Input: part model. Units: mm. Frame: model coordinates. A direction names the side the tool comes from. Round coordinates to 2 decimals unless told otherwise and drop trailing zeros. Loops run counter-clockwise (first coordinate to the right, second up) from the corner with the lowest first, then second, coordinate; pieces in that order, holes last.
(1) Access query for faces 4 (the face through (2, 40, -30)), 5 (the face through (2, 50, -10)), 6 (the face through (2, 3, -20)). Directions: +Z, -Z, +X, -X, +Y, -Y. A direction counts if a zero-diameter tool reaches every point of the face in a straight line with its end or side. Return the directions, or none.
(2) Cut plane D-D, the plane y = 13. Output: boundary loops of the cut face in (x, z), and give its area (3 significant figures).
(3) Cut plane C-C, the plane z = -85. Output: boundary loops of the cut face in (x, y), and give its area (3 significant figures).
(4) Cut plane B-B, the plane z = -15. Output: boundary loops of the cut face in (x, y) (3 decimals).
(5) Line query: line 1 (Y direction, x = 2.95, z = -15) (3 decimals); line 2 (Z direction, x = 2.2, y = 12.5); line 3 (Y direction, x = 4.35, z = -12.5). Output: solid intervals per line, ascending.
(6) Draft query along Z for faces 1 (the face through (2, 0, -85)), 2 (the face through (2, 10, -95)), 3 (the face through (2.535, 8.859, -73.797)). Return one class per face: released by +Z, released by -Z, zero draft, split by the parting line, or undercut.
(7) Cut plane A-A, the plane y = 3. Output: boundary loops of the cut face in (x, z).
(8) First-contact query: pin 1 Ø2.5 at (x, y) = (3, 45.5) entering from -Z; pin 2 Ø3 at (x, z) = (3.5, -83) entering from +Y. Flat tips, straight axial feed; report the tip coordinate or a pass-through.
from build123d import *

# Parameters (mm, degrees)
SKETCH7_R           = 3.225
SKETCH7_R_2         = 4.25
SKETCH7_R_3         = 2.5
SKETCH7_R_4         = 5.25
BOSS_EXTRUDE5_DEPTH = 5
FILLET1_R           = 4
FILLET2_R           = 2


with BuildPart() as part:
    # Sketch7 → Boss-Extrude5 (new body)
    with BuildSketch(Plane(origin=(0, 0, 0), x_dir=(0, 0, -1), z_dir=(1, 0, 0))):
        with BuildLine():
            Line((0, 0), (20, 0))
            Line((20, 0), (20, 10))
            Line((20, 10), (75, 10))
            Line((75, 10), (75, 0))
            Line((75, 0), (95, 0))
            Line((95, 0), (95, 20))
            Line((95, 20), (75, 20))
            ThreePointArc((75, 20), (54.331561409, 24.455232466), (40, 40))
            Line((40, 40), (20, 40))
            Line((20, 40), (20, 50))
            Line((20, 50), (0, 50))
            Line((0, 50), (0, 0))
        make_face()
        with Locations((15, 40)):
            Circle(SKETCH7_R, mode=Mode.SUBTRACT)
        with Locations((15, 10)):
            Circle(SKETCH7_R_2, mode=Mode.SUBTRACT)
        with Locations((40, 27.700051953)):
            Circle(SKETCH7_R_3, mode=Mode.SUBTRACT)
        with Locations((85, 10)):
            Circle(SKETCH7_R_4, mode=Mode.SUBTRACT)
    extrude(amount=BOSS_EXTRUDE5_DEPTH)

    # Fillet1
    fillet1_edges = [part.edges().sort_by_distance(p)[0] for p in [
        (2.5, 10, -75),
        (2.5, 10, -20),
    ]]
    fillet(fillet1_edges, radius=FILLET1_R)

    # Fillet2
    fillet2_edges = [part.edges().sort_by_distance(p)[0] for p in [
        (2.5, 40, -40),
    ]]
    fillet(fillet2_edges, radius=FILLET2_R)


solid = part.part
Reported:
1. face 4: -Z, +X, -X, +Y
1. face 5: +Z, -Z, +X, -X, +Y
1. face 6: +X, -X, -Y
2. outline: (0, -95) - (5, -95) - (5, -89.31) - (0, -89.31) - close; (0, -80.69) - (5, -80.69) - (5, -18.01) - (0, -18.01) - close; (0, -11.99) - (5, -11.99) - (5, 0) - (0, 0) - close
2. area: 402 mm2
3. outline: (0, 0) - (5, 0) - (5, 4.75) - (0, 4.75) - close; (0, 15.25) - (5, 15.25) - (5, 20) - (0, 20) - close
3. area: 47.5 mm2
4. outline: (0, 0) - (5, 0) - (5, 5.75) - (0, 5.75) - close; (0, 14.25) - (5, 14.25) - (5, 36.775) - (0, 36.775) - close; (0, 43.225) - (5, 43.225) - (5, 50) - (0, 50) - close
5. line 1: y = 0 to 5.75, 14.25 to 36.775, 43.225 to 50
5. line 2: z = -95 to -89.62, -80.38 to -18.44, -11.56 to 0
5. line 3: y = 0 to 6.56, 13.44 to 37.96, 42.04 to 50
6. face 1: zero draft
6. face 2: released by -Z
6. face 3: undercut
7. outline: (0, -95) - (5, -95) - (5, -75) - (0, -75) - close; (0, -20) - (5, -20) - (5, 0) - (0, 0) - close
8. pin 1: stops at z = -20
8. pin 2: stops at y = 20
